from build123d import *

# Parameters (mm, degrees)
SKETCH_1_R               = 30
EXTRUDE_1_DEPTH          = 4
SKETCH_2_R               = 28
CUT_EXTRUDE_1_DEPTH      = 1
EXTRUDE_1_2_DEPTH        = 1
PATTERN_CIRCULAR_1_COUNT = 4
SKETCH_4_R               = 10
SKETCH_5_R               = 9
EXTRUDE_START            = -6
SKETCH_6_R               = 4
EXTRUDE_2_DEPTH          = 7
SKETCH_8_R               = 2.5
CUT_EXTRUDE_2_DEPTH      = 4
PATTERN_CIRCULAR_2_COUNT = 4
SKETCH_9_R               = 2
CUT_EXTRUDE_3_DEPTH      = 44.829214027
PATTERN_CIRCULAR_3_COUNT = 4
SKETCH_10_R              = 5
CUT_EXTRUDE_4_DEPTH      = 47.086874487
CUT_EXTRUDE_5_DEPTH      = 47.086874487
PATTERN_CIRCULAR_4_COUNT = 8
SKETCH_12_R              = 3.5
SKETCH_13_R              = 2.9
SKETCH_14_R              = 2
EXTRUDE_3_DEPTH          = 5
SKETCH_15_R              = 1.5
CUT_EXTRUDE_6_DEPTH      = 3
PATTERN_CIRCULAR_5_COUNT = 4


with BuildPart() as part:
    # 草图1 → Extrude 1 (new body)
    with BuildSketch(Plane.XY):
        Circle(SKETCH_1_R)
    extrude(amount=EXTRUDE_1_DEPTH)

    # 草图2 → 切除-拉伸1 (cut)
    with BuildSketch(Plane.XY.offset(4)):
        Circle(SKETCH_2_R)
    extrude(amount=-CUT_EXTRUDE_1_DEPTH, mode=Mode.SUBTRACT)

    # 草图3 → Extrude 1 2 (add)
    with BuildSketch(Plane.XY.offset(3)):
        Polygon((3.00520382, 3.00520382), (-16.793786053, 22.804193693), (-22.804193693, 16.793786053), (-3.00520382, -3.00520382), align=None)
    extrude_1_2 = extrude(amount=EXTRUDE_1_2_DEPTH)

    # 阵列(圆周)1: Extrude 1 2 ×4 about axis
    pattern_circular_1_axis = Axis((0, 0, 0), (0, 0, 1))
    for i in range(1, PATTERN_CIRCULAR_1_COUNT):
        add(extrude_1_2.rotate(pattern_circular_1_axis, i * 360 / PATTERN_CIRCULAR_1_COUNT))

    # 草图4 → 放样1 section 0
    with BuildSketch(Plane.XY.offset(3)):
        Circle(SKETCH_4_R)
    # 草图5 → 放样1 section 1
    with BuildSketch(Plane(origin=(0, 0, 15), x_dir=(-1, 0, 0), z_dir=(0, 0, -1))):
        Circle(SKETCH_5_R)
    loft()

    # 草图6 → 凸台-拉伸2 (add)
    with BuildSketch(Plane.XY.offset(3).offset(EXTRUDE_START)):
        with Locations((0, 22)):
            Circle(SKETCH_6_R)
    extrude_2 = extrude(amount=EXTRUDE_2_DEPTH)

    # 草图8 → 切除-拉伸2 (cut)
    with BuildSketch(Plane(origin=(0, 0, -3), x_dir=(-1, 0, 0), z_dir=(0, 0, -1))):
        with Locations((0, 22)):
            Circle(SKETCH_8_R)
    cut_extrude_2 = extrude(amount=-CUT_EXTRUDE_2_DEPTH, mode=Mode.SUBTRACT)

    # 阵列(圆周)2: 凸台-拉伸2, 切除-拉伸2 ×4 about axis
    pattern_circular_2_axis = Axis((0, 0, 0), (0, 0, 1))
    add([extrude_2.rotate(pattern_circular_2_axis, i * 360 / PATTERN_CIRCULAR_2_COUNT) for i in range(1, PATTERN_CIRCULAR_2_COUNT)])
    add([cut_extrude_2.rotate(pattern_circular_2_axis, i * 360 / PATTERN_CIRCULAR_2_COUNT) for i in range(1, PATTERN_CIRCULAR_2_COUNT)], mode=Mode.SUBTRACT)

    # 草图9 → 切除-拉伸3 (cut, through all)
    with BuildSketch(Plane.XY.offset(4)):
        with Locations((-15.556349269, 15.556349103)):
            Circle(SKETCH_9_R)
    cut_extrude_3 = extrude(amount=-CUT_EXTRUDE_3_DEPTH, mode=Mode.SUBTRACT)

    # 阵列(圆周)3: 切除-拉伸3 ×4 about axis
    pattern_circular_3_axis = Axis((0, 0, 0), (0, 0, 1))
    for i in range(1, PATTERN_CIRCULAR_3_COUNT):
        add(cut_extrude_3.rotate(pattern_circular_3_axis, i * 360 / PATTERN_CIRCULAR_3_COUNT), mode=Mode.SUBTRACT)

    # 草图10 → 切除-拉伸4 (cut, through all)
    with BuildSketch(Plane.XY.offset(15)):
        Circle(SKETCH_10_R)
    extrude(amount=-CUT_EXTRUDE_4_DEPTH, mode=Mode.SUBTRACT)

    # 草图11 → 切除-拉伸5 (cut, through all)
    with BuildSketch(Plane.XY.offset(15)):
        with BuildLine():
            Line((1, -5.916079783), (1, 5.916079783))
            ThreePointArc((1, 5.916079783), (0, 6), (-1, 5.916079783))
            Line((-1, 5.916079783), (-1, -5.916079783))
            ThreePointArc((-1, -5.916079783), (0, -6), (1, -5.916079783))
        make_face()
    cut_extrude_5 = extrude(amount=-CUT_EXTRUDE_5_DEPTH, mode=Mode.SUBTRACT)

    # 阵列(圆周)4: 切除-拉伸5 ×8 about axis
    pattern_circular_4_axis = Axis((0, 0, 0), (0, 0, 1))
    for i in range(1, PATTERN_CIRCULAR_4_COUNT):
        add(cut_extrude_5.rotate(pattern_circular_4_axis, i * 360 / PATTERN_CIRCULAR_4_COUNT), mode=Mode.SUBTRACT)

    # 草图12 → 放样2 section 0
    with BuildSketch(Plane(origin=(0, 0, 0), x_dir=(-1, 0, 0), z_dir=(0, 0, -1))):
        with Locations((-15.556349186, 15.556349186)):
            Circle(SKETCH_12_R)
    # 草图13 → 放样2 section 1
    with BuildSketch(Plane(origin=(0, 0, -17), x_dir=(-1, 0, 0), z_dir=(0, 0, -1))):
        with Locations((-15.556349186, 15.556349186)):
            Circle(SKETCH_13_R)
    loft_2 = loft()

    # 草图14 → 凸台-拉伸3 (add)
    with BuildSketch(Plane(origin=(0, 0, -17), x_dir=(-1, 0, 0), z_dir=(0, 0, -1))):
        with Locations(Location((-15.556349186, 15.556349186, 0), (0, 0, 179.999997613))):
            Circle(SKETCH_14_R)
    extrude_3 = extrude(amount=EXTRUDE_3_DEPTH)

    # 草图15 → 切除-拉伸6 (cut)
    with BuildSketch(Plane(origin=(0, 0, -22), x_dir=(-1, 0, 0), z_dir=(0, 0, -1))):
        with Locations((-15.556349186, 15.556349186)):
            Circle(SKETCH_15_R)
    cut_extrude_6 = extrude(amount=-CUT_EXTRUDE_6_DEPTH, mode=Mode.SUBTRACT)

    # 阵列(圆周)5: 放样2, 凸台-拉伸3, 切除-拉伸6 ×4 about axis
    pattern_circular_5_axis = Axis((0, 0, 0), (0, 0, 1))
    add([loft_2.rotate(pattern_circular_5_axis, i * 360 / PATTERN_CIRCULAR_5_COUNT) for i in range(1, PATTERN_CIRCULAR_5_COUNT)])
    add([extrude_3.rotate(pattern_circular_5_axis, i * 360 / PATTERN_CIRCULAR_5_COUNT) for i in range(1, PATTERN_CIRCULAR_5_COUNT)])
    add([cut_extrude_6.rotate(pattern_circular_5_axis, i * 360 / PATTERN_CIRCULAR_5_COUNT) for i in range(1, PATTERN_CIRCULAR_5_COUNT)], mode=Mode.SUBTRACT)


solid = part.part
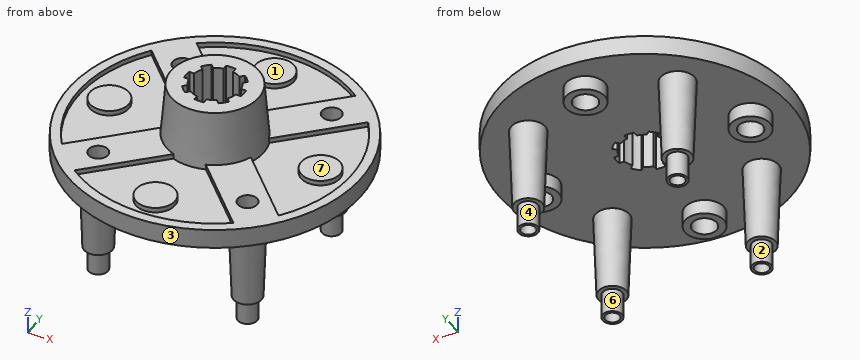
The model under review builds one solid part; all positions refer to its coordinate system, in mm. Face numbers are marked on the shaded views. A direction names the side the tool comes from. Give positions to 0.01 mm unless a question says otherwise; leave off trailing zeros. Order: outer loops, then holes, each group sorted by start corner. A loop starts at its lowest first (then second) coordinate and runs counter-clockwise, first axis right, second up. Notation, with made-up numbers: M -22.75,54 L -16.75,54 A29 cw -16.75,80 Z; hole C 22.5,40.25 d5. An arc over 180 degrees is marked long. Answer in a Markdown table with one row per item. Add a question column.
1. For pin 1 Ø2 at (x, y) = (-16.5, 15.5) entering from +Z; pin 2 Ø2.5 at (x, y) = (-0.5, -21) entering from -Z; pin 3 Ø0.8 at (y, z) = (5.5, 4) entering from +X, all flat-tipped, find the tip position at first contact; note any pin that passes through.
2. To check wall thickness, follow line 1 along Z through (x, y) = (14, 5.5); line 2 along Y through (x, z) = (-22, -0.8); line 3 along Z through (x, y) = (-20.5, 3). State the ranges of each line that lie inside material, in increasing order.
3. Add section C-C on z = -6. State the section outline as (x, y) points.
4. Machinability: for the marked faces 5, 6 and 7, which of the approach directions +Z, -Z, +X, -X, +Y, -Y give a long, thin tool a straight path to every point of the face, cutting with its end or side? Answer none if there is none.
5. Mouldability with a two-part tool opening along Y and no side actions: class the marked faces 1, 2, 3 and 4 as released by +Y, released by -Y, zero draft, split by the parting line, or undercut.
6. Add section A-A on z = -13. State the section outline as (x, y) points, plus the area to 3 significant figures.
7. Add section B-B on x = 20.5. State the section outline as (y, z) points.
The answers:
| question | item | result |
|---|---|---|
| 1 | pin 1 | z = 0 |
| 1 | pin 2 | z = 1 |
| 1 | pin 3 | x = 29.56 |
| 2 | line 1 | 0 to 3 |
| 2 | line 2 | -4 to -2.5, 2.5 to 4 |
| 2 | line 3 | -3 to 4 |
| 3 | outline | C -15.56,-15.56 d6.58; C -15.56,15.56 d6.58; C 15.56,-15.56 d6.58; C 15.56,15.56 d6.58 |
| 4 | face 5 | +Z |
| 4 | face 6 | -Z |
| 4 | face 7 | +Z, +X, +Y, -Y |
| 5 | face 1 | zero draft |
| 5 | face 2 | undercut |
| 5 | face 3 | split by the parting line |
| 5 | face 4 | undercut |
| 6 | outline | C -15.56,-15.56 d6.08; C -15.56,15.56 d6.08; C 15.56,-15.56 d6.08; C 15.56,15.56 d6.08 |
| 6 | area | 116 mm2 |
| 7 | outline | M -21.9,0 L -3.71,0 L -3.71,-3 L -2,-3 L -2,1 L 2,1 L 2,-3 L 3.71,-3 L 3.71,0 L 21.9,0 L 21.9,4 L 14.49,4 L 14.49,3 L 3.71,3 L 3.71,4 L -3.71,4 L -3.71,3 L -14.49,3 L -14.49,4 L -21.9,4 Z |
